```python
from build123d import *

# Parameters (mm, degrees)
F0_R     = 100
F0_R_2   = 85
F1_DEPTH = 50
F0_R_3   = 120
F2_DEPTH = 20
F3_R     = 10


with BuildPart() as f1:
    # F0 (on Top) → F1 (new body)
    with BuildSketch(Plane.XY):
        Circle(F0_R)
        Circle(F0_R_2, mode=Mode.SUBTRACT)
    extrude(amount=-F1_DEPTH)

    # F0 (on Top) → F2 (join)
    with BuildSketch(Plane.XY):
        Circle(F0_R_3)
        Circle(F0_R, mode=Mode.SUBTRACT)
        Circle(F0_R)
        Circle(F0_R_2, mode=Mode.SUBTRACT)
    extrude(amount=F2_DEPTH)

    # F3
    f3_edges = [f1.edges().sort_by_distance(p)[0] for p in [
        (-120, 0, 20),
    ]]
    fillet(f3_edges, radius=F3_R)


solid = f1.part
```
The listing builds one solid part. Answer for the finished solid, in the listing's coordinates (mm). A direction names the side the tool comes from. Coordinates: 2 decimals unless noted, no trailing zeros. Loops run counter-clockwise (first coordinate to the right, second up) from the corner with the lowest first, then second, coordinate; pieces in that order, holes last. Notation, with made-up numbers: (-7, 51) -> (47, 51) arc R17 cw to (47, 60) -> close; hole circle Ø11 at (54, -3). An arc over 180 degrees is marked (long way). Return JSON: item names as keys, results as strings. Group by question number.
(1) Find the intervals of material crossed by probe 1 along Y at (x, z) = (0, 1); probe 2 along Y at (x, z) = (0, -6); probe 3 along X at (y, z) = (-48, 13.5), in increasing order. Write a range as from..to.
(2) A cutting plane is placed at A-A on x = 0. Write down the section's boundary in (y, z), and give its area (3 significant figures).
(3) Given pin 1 Ø5 at (x, z) = (-31, -14.5) entering from -Y; pin 2 Ø6 at (x, z) = (-57.5, -25.5) entering from -Y; pin 3 Ø8 at (y, z) = (95.5, -16.5) entering from -X, each flat-ended and moving along its own axis, determine where each tip first touches the part or whether it passes through.
(4) A cutting plane is placed at C-C on z = -8.5. Write down the section's boundary in (x, y), and give its area (3 significant figures).
(5) Determine the mould class of faces 3 (the cylindrical face through (-119.884, 5.276, 4.93)), 4 (the flat face through (-45, -74, -50)), 5 (the cylindrical face through (-67.453, -51.721, -15.49)) for opening direction Y: released by +Y, released by -Y, zero draft, split by the parting line, or undercut.
(6) Which of the six approach directions +Z, -Z, +X, -X, +Y, -Y give full straight-line access (tool end or side, diameter ignored) to faces 1 (the flat face through (-27, 98, 0)), 2 (the flat face through (57, -65, 20))?
The answers:
{
 "1": {"probe 1": "y = -120..-85, 85..120", "probe 2": "y = -100..-85, 85..100", "probe 3": "x = -109.29..-70.15, 70.15..109.29"},
 "2": {"outline": "(-120, 0) -> (-100, 0) -> (-100, -50) -> (-85, -50) -> (-85, 20) -> (-110, 20) arc R10 ccw to (-120, 10) -> close; (85, -50) -> (100, -50) -> (100, 0) -> (120, 0) -> (120, 10) arc R10 ccw to (110, 20) -> (85, 20) -> close", "area": "2,860 mm^2"},
 "3": {"pin 1": "stops at y = -95.85", "pin 2": "stops at y = -83.84", "pin 3": "stops at x = -40.35"},
 "4": {"outline": "circle Ø200 at (0, 0); hole circle Ø170 at (0, 0)", "area": "8,720 mm^2"},
 "5": {"face 3": "split by the parting line", "face 4": "zero draft", "face 5": "undercut"},
 "6": {"face 1": "-Z", "face 2": "+Z, +X, -X, +Y, -Y"}
}
